```python
from build123d import *

# Parameters (mm, degrees)
F1_R     = 4
F2_DEPTH = 4.06
F3_D     = 5
F5_DEPTH = 25.4
F7_DEPTH = 25.4
F9_DEPTH = 0.127


with BuildPart() as f2:
    # F1 (on Top) → F2 (new body)
    with BuildSketch(Plane.XY):
        with BuildLine():
            Line((26, 14.04), (26, 21))
            Line((26, 21), (-33, 21))
            Line((-33, 21), (-33, -21))
            Line((-33, -21), (26, -21))
            Line((26, -21), (26, -11.5))
            Line((26, -11.5), (33, -11.5))
            Line((33, -11.5), (33, 11.5))
            Line((33, 11.5), (28.54, 11.5))
            ThreePointArc((28.54, 11.5), (26.7439487758, 12.2439487758), (26, 14.04))
        make_face()
        with Locations((19, -15.5)):
            Circle(F1_R, mode=Mode.SUBTRACT)
        with Locations((19, 15.5)):
            Circle(F1_R, mode=Mode.SUBTRACT)
    extrude(amount=F2_DEPTH)

    # F3 (through all)
    with Locations(Plane(origin=(0, 0, 0), x_dir=(1, 0, 0), z_dir=(0, 0, -1))):
        with Locations((-11, 0)):
            Hole(F3_D / 2)

    # F4 (on face) → F5 (cut)
    with BuildSketch(Plane(origin=(0, 0, 0), x_dir=(1, 0, 0), z_dir=(0, 0, -1))):
        Polygon((-23.7, -20.20625), (-23.7, -21), (1.7, -21), (1.7, -20.20625), (-3.0625, -18.7775), (-18.9375, -18.7775), align=None)
        Polygon((1.7, 21), (-23.7, 21), (-23.7, 20.20625), (-18.9375, 18.7775), (-3.0625, 18.7775), (1.7, 20.20625), align=None)
    extrude(amount=-F5_DEPTH, mode=Mode.SUBTRACT)

    # F6 (on face) → F7 (cut)
    with BuildSketch(Plane.XY.offset(4.06)):
        with BuildLine():
            ThreePointArc((-22.6000877886, 11.9506443438), (-23.5215163343, 9.4190402209), (-20.9899122114, 8.4976116752))
            Line((-20.9899122114, 8.4976116752), (-17.6239996184, 10.067162494))
            Line((-17.6239996184, 10.067162494), (-4.3760003816, 10.067162494))
            Line((-4.3760003816, 10.067162494), (-1.0100877886, 8.4976116752))
            ThreePointArc((-1.0100877886, 8.4976116752), (1.3090855116, 4.5270480494), (2.1151725179, 0))
            ThreePointArc((2.1151725179, 0), (1.3090855116, -4.5270480494), (-1.0100877886, -8.4976116752))
            Line((-1.0100877886, -8.4976116752), (-4.3760003816, -10.067162494))
            Line((-4.3760003816, -10.067162494), (-17.6239996184, -10.067162494))
            Line((-17.6239996184, -10.067162494), (-20.9899122114, -8.4976116752))
            ThreePointArc((-20.9899122114, -8.4976116752), (-23.5215163343, -9.4190402209), (-22.6000877886, -11.9506443438))
            Line((-22.6000877886, -11.9506443438), (-18.4686562831, -13.877162494))
            Line((-18.4686562831, -13.877162494), (-3.5313437169, -13.877162494))
            Line((-3.5313437169, -13.877162494), (1.3034740029, -11.6226499654))
            ThreePointArc((1.3034740029, -11.6226499654), (4.7273628563, -6.253920558), (5.9251725179, 0))
            ThreePointArc((5.9251725179, 0), (4.7273628563, 6.253920558), (1.3034740029, 11.6226499654))
            Line((1.3034740029, 11.6226499654), (-3.5313437169, 13.877162494))
            Line((-3.5313437169, 13.877162494), (-18.4686562831, 13.877162494))
            Line((-18.4686562831, 13.877162494), (-22.6000877886, 11.9506443438))
        make_face()
    extrude(amount=-F7_DEPTH, mode=Mode.SUBTRACT)

    # F8 (on face) → F9 (cut)
    with BuildSketch(Plane.XY.offset(4.06)):
        Polygon((13.85, 21), (-23.7, 21), (-23.7, 10.067162494), (2.1151725179, 10.067162494), (2.1151725179, -10.067162494), (-23.7, -10.067162494), (-23.7, -21), (13.85, -21), (13.85, 0), align=None)
    extrude(amount=-F9_DEPTH, mode=Mode.SUBTRACT)


solid = f2.part
```
The model under review builds one solid part; all positions refer to its coordinate system, in mm. A direction names the side the tool comes from. Round coordinates to 2 decimals unless told otherwise and drop trailing zeros. Loops run counter-clockwise (first coordinate to the right, second up) from the corner with the lowest first, then second, coordinate; pieces in that order, holes last.
Item 1: Take a section at D-D (x = 4.5). Write out the cut boundary in (y, z), then the cut area to 3 significant figures.
Determined:
outline: (-21, 0) - (-6.8, 0) - (-6.8, 3.93) - (-21, 3.93) - close; (6.8, 0) - (21, 0) - (21, 3.93) - (6.8, 3.93) - close
area: 112 mm2
Item 2: For faces 1 (the face through (-23.7, -20.4, 2.6)), 2 (the face through (-2.67, -9.27, 2.06)), 3 (the face through (-21.35, -19.5, 1.94)), list the 3-axis set-ups (+Z, -Z, +X, -X, +Y, -Y) from which the entire face can be reached by the end or side of a thin tool; tool diameter is ignored.
Determined:
face 1: +Z, -Y
face 2: +Z, -Z
face 3: +Z, -Z, -Y
Item 3: Take a section at A-A (x = -11). Write out the cut boundary in (y, z).
Determined:
outline: (-18.78, 0) - (-13.88, 0) - (-13.88, 3.93) - (-18.78, 3.93) - close; (-10.07, 0) - (-2.5, 0) - (-2.5, 4.06) - (-10.07, 4.06) - close; (2.5, 0) - (10.07, 0) - (10.07, 4.06) - (2.5, 4.06) - close; (13.88, 0) - (18.78, 0) - (18.78, 3.93) - (13.88, 3.93) - close
Item 4: Clearance check with flat-ended pins moving along their axes: pin 1 Ø2 at (x, z) = (-13.5, 1.5) entering from +Y; pin 2 Ø1 at (x, y) = (1, -14) entering from +Z; pin 3 Ø1.2 at (y, z) = (18, 2.5) entering from +X. State where each tip first meets the part, or that it passes through.
Determined:
pin 1: stops at y = 18.78
pin 2: stops at z = 3.93
pin 3: stops at x = 26
Item 5: Take a section at B-B (y = -15.5). Write out the cut boundary in (x, z), then the cut area to 3 significant figures.
Determined:
outline: (-33, 0) - (15, 0) - (15, 4.06) - (13.85, 4.06) - (13.85, 3.93) - (-23.7, 3.93) - (-23.7, 4.06) - (-33, 4.06) - close; (23, 0) - (26, 0) - (26, 4.06) - (23, 4.06) - close
area: 202 mm2
Item 6: Mouldability with a two-part tool opening along Y and no side actions: class faces 4 (the face through (29, -11.5, 2)), 5 (the face through (31, 11.5, 2)), 6 (the face through (-19.283, -9.293, 2.058)) as released by +Y, released by -Y, zero draft, split by the parting line, or undercut.
Determined:
face 4: released by -Y
face 5: released by +Y
face 6: undercut
Item 7: For line 1 (Y direction, x = 19, z = 1.85); line 2 (Y direction, x = -17.5, z = 1.25); line 3 (Y direction, x = -10.5, z = 1.15), list the stretches that pass through material, from the lowest coordinate up.
Determined:
line 1: y = -21 to -19.5, -11.5 to 11.5, 19.5 to 21
line 2: y = -18.78 to -13.88, -10.07 to 10.07, 13.88 to 18.78
line 3: y = -18.78 to -13.88, -10.07 to -2.45, 2.45 to 10.07, 13.88 to 18.78
Item 8: Take a section at C-C (x = 19). Write out the cut boundary in (y, z), then the cut area to 3 significant figures.
Determined:
outline: (-21, 0) - (-19.5, 0) - (-19.5, 4.06) - (-21, 4.06) - close; (-11.5, 0) - (11.5, 0) - (11.5, 4.06) - (-11.5, 4.06) - close; (19.5, 0) - (21, 0) - (21, 4.06) - (19.5, 4.06) - close
area: 106 mm2
